```python
from build123d import *

# Parameters (mm, degrees)
F0_W      = 600
F0_H      = 600
F1_DEPTH  = 20
F2_W      = 50
F2_H      = 20
F3_W      = 50
F3_H      = 20
F8_DEPTH  = 50.8
F4_W      = 50
F4_H      = 20
F5_W      = 50
F5_H      = 20
F11_DEPTH = 50.8
F6_W      = 50
F6_H      = 20
F7_W      = 50
F7_H      = 20
F12_DEPTH = 50.8
F9_W      = 50
F9_H      = 20
F10_W     = 50
F10_H     = 20
F13_DEPTH = 50.8


# Not quite as in the source:
# - a feature names something its author has since deleted; it is built from what else it names


with BuildPart() as f1:
    # F0 (on Top) → F1 (new body)
    with BuildSketch(Plane.XY):
        with Locations((-57.8414618969, -13.7785196304)):
            Rectangle(F0_W, F0_H)
        Polygon((-257.8414618969, 111.6214803696), (-257.8414618969, 186.2214803696), (-183.2414618969, 186.2214803696), (-183.2414618969, 236.2214803696), (-157.8414618969, 236.2214803696), (-132.4414618969, 236.2214803696), (-132.4414618969, 186.2214803696), (16.7585381031, 186.2214803696), (16.7585381031, 236.2214803696), (67.5585381031, 236.2214803696), (67.5585381031, 186.2214803696), (142.1585381031, 186.2214803696), (142.1585381031, 111.6214803696), (192.1585381031, 111.6214803696), (192.1585381031, 60.8214803696), (142.1585381031, 60.8214803696), (142.1585381031, -88.3785196304), (192.1585381031, -88.3785196304), (192.1585381031, -139.1785196304), (142.1585381031, -139.1785196304), (142.1585381031, -213.7785196304), (67.5585381031, -213.7785196304), (67.5585381031, -263.7785196304), (16.7585381031, -263.7785196304), (16.7585381031, -213.7785196304), (-132.4414618969, -213.7785196304), (-132.4414618969, -263.7785196304), (-183.2414618969, -263.7785196304), (-183.2414618969, -213.7785196304), (-257.8414618969, -213.7785196304), (-257.8414618969, -139.1785196304), (-307.8414618969, -139.1785196304), (-307.8414618969, -88.3785196304), (-257.8414618969, -88.3785196304), (-257.8414618969, -13.7785196304), (-257.8414618969, 60.8214803696), (-307.8414618969, 60.8214803696), (-307.8414618969, 111.6214803696), align=None, mode=Mode.SUBTRACT)
    extrude(amount=F1_DEPTH)

    # F2 (on face) + F3 (on face) → F8 (join)
    with BuildSketch(Plane.XZ.offset(88.3785196304)):
        Polygon((-307.8414618969, 20), (-257.8414618969, 20), (-307.8414618969, 120), align=None)
        with Locations((-282.8414618969, 10)):
            Rectangle(F2_W, F2_H)
    with BuildSketch(Plane.XZ.offset(-111.6214803696)):
        Polygon((-307.8414618969, 20), (-257.8414618969, 20), (-307.8414618969, 120), align=None)
        with Locations((-282.8414618969, 10)):
            Rectangle(F3_W, F3_H)
    extrude(amount=F8_DEPTH)

    # F4 (on face) + F5 (on face) → F11 (join)
    with BuildSketch(Plane(origin=(-132.4414618969, 0, 0), x_dir=(0, -1, 0), z_dir=(-1, 0, 0))):
        Polygon((-236.2214803696, 20), (-186.2214803696, 20), (-236.2214803696, 120), align=None)
        with Locations((-211.2214803696, 10)):
            Rectangle(F4_W, F4_H)
    with BuildSketch(Plane(origin=(67.5585381031, 0, 0), x_dir=(0, -1, 0), z_dir=(-1, 0, 0))):
        with Locations((-211.2214803696, 10)):
            Rectangle(F5_W, F5_H)
        Polygon((-236.2214803696, 20), (-186.2214803696, 20), (-236.2214803696, 120), align=None)
    extrude(amount=F11_DEPTH)

    # F6 (on face) + F7 (on face) → F12 (join)
    with BuildSketch(Plane(origin=(0, 60.8214803696, 0), x_dir=(-1, 0, 0), z_dir=(0, 1, 0))):
        with Locations((-167.1585381031, 10)):
            Rectangle(F6_W, F6_H)
        Polygon((-192.1585381031, 20), (-142.1585381031, 20), (-192.1585381031, 120), align=None)
    with BuildSketch(Plane(origin=(0, -139.1785196304, 0), x_dir=(-1, 0, 0), z_dir=(0, 1, 0))):
        with Locations((-167.1585381031, 10)):
            Rectangle(F7_W, F7_H)
        Polygon((-192.1585381031, 20), (-142.1585381031, 20), (-192.1585381031, 120), align=None)
    extrude(amount=F12_DEPTH)

    # F9 (on face) + F10 (on face) → F13 (join)
    with BuildSketch(Plane.YZ.offset(16.7585381031)):
        with Locations((-238.7785196304, 10)):
            Rectangle(F9_W, F9_H)
        Polygon((-263.7785196304, 20), (-213.7785196304, 20), (-263.7785196304, 120), align=None)
    with BuildSketch(Plane.YZ.offset(-183.2414618969)):
        with Locations((-238.7785196304, 10)):
            Rectangle(F10_W, F10_H)
        Polygon((-263.7785196304, 20), (-213.7785196304, 20), (-263.7785196304, 120), align=None)
    extrude(amount=F13_DEPTH)


solid = f1.part
```
Design review of the part built by this model. Coordinates are the model's own, in mm. A direction names the side the tool comes from. Coordinates: 2 decimals unless noted, no trailing zeros. Loops run counter-clockwise (first coordinate to the right, second up) from the corner with the lowest first, then second, coordinate; pieces in that order, holes last. Notation, with made-up numbers: M 30.25,-1 L 45.25,-1 A25 cw 45.25,20 Z; hole C -15,0.5 d2. An arc over 180 degrees is marked long. One line per question, with ' | ' between items.
(1) Draft analysis for pull direction Y (two halves, no side actions). For faces 5 (the face through (-158.2, -238.43, 69.3)), 6 (the face through (-294, 111.621, 48)), 7 (the face through (67.559, 223, 48)), 8 (the face through (42, -263.779, 71)), state which applies: released by +Y, released by -Y, zero draft, split by the parting line, or undercut.
Filled in:
face 5: undercut | face 6: released by +Y | face 7: zero draft | face 8: released by -Y
(2) For pin 1 Ø15 at (y, z) = (-251, 68) entering from -X; pin 2 Ø15 at (x, z) = (35, 94.5) entering from -Y; pin 3 Ø12 at (y, z) = (29.5, 21.5) entering from -X; pin 4 Ø25 at (y, z) = (-240.5, 85) entering from +X, all flat-tipped, find the tip position at first contact; note any pin that passes through.
Filled in:
pin 1: stops at x = -183.24 | pin 2: stops at y = -263.78 | pin 3: stops at x = -357.84 | pin 4: stops at x = 67.56
(3) We need section B-B (x = 35.5). Give the boundary of the cut face in (y, z), and give its area (3 significant figures).
Filled in:
outline: M -313.78,0 L -213.78,0 L -213.78,20 L -263.78,120 L -263.78,20 L -313.78,20 Z; M 186.22,0 L 286.22,0 L 286.22,20 L 236.22,20 L 236.22,120 L 186.22,20 Z | area: 9,000 mm^2
(4) We need section A-A (y = 95.5). Give the boundary of the cut face in (x, z).
Filled in:
outline: M -357.84,0 L -257.84,0 L -257.84,20 L -307.84,120 L -307.84,20 L -357.84,20 Z; M 142.16,0 L 242.16,0 L 242.16,20 L 192.16,20 L 192.16,120 L 142.16,20 Z
(5) We need section D-D (y = 160). Give the boundary of the cut face in (x, z).
Filled in:
outline: M -357.84,0 L -257.84,0 L -257.84,20 L -357.84,20 Z; M 142.16,0 L 242.16,0 L 242.16,20 L 142.16,20 Z
(6) We need section C-C (z = 98.5). Count the separate pieces of the cut face and the enclosed holes in it, and give its area (3 significant figures).
Filled in:
separate pieces: 8 | enclosed holes: 0 | area: 4,370 mm^2
(7) Machinability: for faces 1 (the face through (-294, -88.379, 48)), 2 (the face through (-294, -139.179, 48)), 3 (the face through (16.759, -250, 48)), 4 (the face through (-307.841, 87, 71)), which of the approach directions +Z, -Z, +X, -X, +Y, -Y give a long, thin tool a straight path to every point of the face, cutting with its end or side? Answer none if there is none.
Filled in:
face 1: +Z, +X, -X | face 2: +Z, +X, -X, -Y | face 3: +Z, +Y, -Y | face 4: +Z, -X, +Y, -Y
(8) Wall thickness on probe 1 along Y at (x, z) = (-93.5, 19); probe 2 along X at (y, z) = (209, 26.5); probe 3 along Y at (x, z) = (167, 38): over which ranges is each line inside the solid? List them lowest first.
Filled in:
probe 1: y = -313.78 to -213.78, 186.22 to 286.22 | probe 2: x = -183.24 to -132.44, 16.76 to 67.56 | probe 3: y = -139.18 to -88.38, 60.82 to 111.62
